Could you check a few things on this model? Use its own coordinates, in mm. Give positions to 0.01 mm unless a question says otherwise; leave off trailing zeros. Loops run counter-clockwise (first coordinate to the right, second up) from the corner with the lowest first, then second, coordinate; pieces in that order, holes last. Notation, with made-up numbers: (79.25, -19.5) -> (121.25, -19.5) arc R25 ccw to (121.25, 14.5) -> close; hole circle Ø10 at (48.25, 5.25). An arc over 180 degrees is marked (long way). Write item = value, one per line. Start each with the question number.
1) I want a section at A-A (z = 0). List the corners of the cut face in (x, y) for me.
2) If we mould it in two halves opening along X, with no side actions, what happens to faces 1 (the face through (-7.5, 0.3, 0.1)), 2 (the face through (-4.1, 0.3, 0)), 3 (the face through (0.972, 0.296, 1.687))? For each: +X half, -X half, draft (parallel to the pull), parting line (faces both ways), or undercut.
3) I want a section at D-D (z = -2.05). List the corners of the cut face in (x, y) for me, and give its area (3 significant figures).
4) I want a section at C-C (x = 5). List the corners of the cut face in (y, z) for me, and give its area (3 significant figures).
5) I want a section at B-B (y = 0.2). List the corners of the cut face in (x, z) for me.
6) I need wall thicknesses on probe 1 along Z at (x, y) = (-5, 0.2); probe 2 along Y at (x, z) = (1.5, -0.15); probe 3 along Z at (x, y) = (-5.75, 0.55). Which ranges of each line are inside material? Lowest first, please. Write a range as from..to.
7) I'm going to push flat-ended pins straight in: pin 1 Ø1.5 at (x, z) = (-4, 1) entering from -Y; pin 2 Ø1 at (x, z) = (4, 2) entering from -Y. Where does each tip first touch, or does it pass through?
Autodesk Inventor part; units mm, degrees
ref_plane "YZ Plane" through (0, 0, 0) normal (1, 0, 0) x (0, 1, 0)
ref_plane "XZ Plane" through (0, 0, 0) normal (0, 1, 0) x (-1, 0, 0)
ref_plane "XY Plane" through (0, 0, 0) normal (0, 0, 1) x (1, 0, 0)
sketch "Sketch2" plane through (0, 0, 0) normal (0, 1, 0) x (-1, 0, 0)
  line L0 (-7.5, 0.85) -> (-7.5, -0.85)
  line L1 (1, -2.5) -> (5, -2.5)
  line L2 (7.5, 2.5) -> (-7.5, -2.5) construction
  line L3 (-7.5, 2.5) -> (7.5, -2.5) construction
  arc A0 (5, -2.5) -> (5, 2.5) centre (5, 0) ccw
  circle A1 centre (5, 0) radius 0.9
  line L4 (-3, 0.85) -> (-7.5, 0.85)
  line L5 (-7.5, 0.85) -> (-7.5, -0.85)
  line L6 (-7.5, -0.85) -> (-3, -0.85)
  line L7 (1, 2.5) -> (-3, 0.85)
  line L8 (-3, -0.85) -> (1, -2.5)
  line L9 (5, 2.5) -> (1, 2.5)
  point P0 (0, 0)
  dimension "d3" = 1.8
extrude "Extrusion1" add sketch "Sketch2" along normal blind 0.6
sketch "Sketch3" plane through (0, 0, 0) normal (0, -1, 0) x (1, 0, 0)
  line L0 (-2.413, -1.1278) -> (-2.413, 1.9227) construction
  line L1 (-2.413, 1.9227) -> (-0.0196, 1.9227) construction
  line L2 (-0.0196, 1.9227) -> (-0.0196, -1.1278) construction
  line L3 (-0.0196, -1.1278) -> (-2.413, -1.1278) construction
  line L4 (-2.1487, 1.1916) -> (-2.1487, -1.1599)
  line L5 (-2.1487, -1.1599) -> (-2.413, -1.1599)
  line L6 (-2.413, -1.1599) -> (-2.413, 1.1916)
  line L7 (-2.413, 1.1916) -> (-2.1487, 1.1916)
  point P0 (0, 0)
extrude "Extrusion2" add sketch "Sketch3" along normal blind 0.1
properties part number "Negative Pin" material "Copper, Alloy"
Answer list:
q1.outline = (-7.5, 0) -> (-5.9, 0) -> (-5.9, 0.6) -> (-7.5, 0.6) -> close; (-4.1, 0) -> (-2.41, 0) -> (-2.41, -0.1) -> (-2.15, -0.1) -> (-2.15, 0) -> (7.5, 0) -> (7.5, 0.6) -> (-4.1, 0.6) -> close
q2.face_1 = -X half
q2.face_2 = undercut
q2.face_3 = +X half
q3.outline = (-6.43, 0) -> (0.09, 0) -> (0.09, 0.6) -> (-6.43, 0.6) -> close
q3.area = 3.91 mm^2
q4.outline = (0, -0.85) -> (0.6, -0.85) -> (0.6, 0.85) -> (0, 0.85) -> close
q4.area = 1.02 mm^2
q5.outline = (-5, -2.5) -> (-1, -2.5) -> (3, -0.85) -> (7.5, -0.85) -> (7.5, 0.85) -> (3, 0.85) -> (-1, 2.5) -> (-5, 2.5) arc R2.5 ccw to start; hole circle Ø1.8 at (-5, 0)
q6.probe_1 = -2.5..-0.9, 0.9..2.5
q6.probe_2 = 0..0.6
q6.probe_3 = -2.38..-0.5, 0.5..2.38
q7.pin_1 = 0
q7.pin_2 = through
